```python
from build123d import *

# Parameters (mm, degrees)
S_BOX1_W       = 20
S_BOX1_H       = 2.5
BOSS_1_DEPTH   = 42
S_BOX2_W       = 30.4
S_BOX2_H       = 17
BOSS_2_DEPTH   = 27.6
S_CUT3_W       = 30.6
S_CUT3_H       = 13
POCKET_3_DEPTH = 23.6
S_HOLE4_R      = 1.5
HOLE_4_DEPTH   = 2.7


with BuildPart() as part:
    # S_box1 → Boss_1 (new body)
    with BuildSketch(Plane.XY.offset(-34)):
        with Locations((0, -2.75)):
            Rectangle(S_BOX1_W, S_BOX1_H)
    extrude(amount=BOSS_1_DEPTH)

    # S_box2 → Boss_2 (add)
    with BuildSketch(Plane.XY.offset(-35.4)):
        with Locations((-3.8, -10)):
            Rectangle(S_BOX2_W, S_BOX2_H)
    extrude(amount=BOSS_2_DEPTH)

    # S_cut3 → Pocket_3 (cut)
    with BuildSketch(Plane.XY.offset(-33.4)):
        with Locations((-3.8, -10)):
            Rectangle(S_CUT3_W, S_CUT3_H)
    extrude(amount=POCKET_3_DEPTH, mode=Mode.SUBTRACT)

    # S_hole4 → Hole_4 (cut)
    with BuildSketch(Plane(origin=(0, -4.1, 0), x_dir=(1, 0, 0), z_dir=(0, 1, 0))):
        with Locations(Location((0, 0, 0), (0, 0, 90))):
            Circle(S_HOLE4_R)
    extrude(amount=HOLE_4_DEPTH, mode=Mode.SUBTRACT)


solid = part.part
```
Geometry check sheet. Reference: the model listing, model coordinates, mm. A direction names the side the tool comes from. Round coordinates to 2 decimals unless told otherwise and drop trailing zeros. Loops run counter-clockwise (first coordinate to the right, second up) from the corner with the lowest first, then second, coordinate; pieces in that order, holes last. Notation, with made-up numbers: M 78,-40 L 136,-40 A17 ccw 136,-8 Z; hole C 25,27 d4. An arc over 180 degrees is marked long. Return JSON: item names as keys, results as strings. Group by question number.
(1) Scan lines: line 1 along X through (y, z) = (-2, 0); line 2 along Z through (x, y) = (6, -7); line 3 along Y through (x, z) = (1, -18). Record each from-to range of solid material in increasing order. Write a range as [from, to].
(2) Section check A-A, the plane x = 0. Enter the section's corners in (y, z).
(3) Go/stop test with flat-tipped pins: pin 1 (17.5 mm diameter, centred on x = -4, z = 3.5, fed in from -Y); pin 2 (5 mm diameter, centred on x = -8, y = -10, fed in from +Z); pin 3 (0.8 mm diameter, centred on y = -3, z = -1.5, fed in from -X). Record where each tip stops, or that it passes through.
(4) Set-up check for faces 5 (the face through (10, -3, 0)), 6 (the face through (0, -4, 2)), 7 (the face through (-4, -10, -33.4)): record each of +Z, -Z, +X, -X, +Y, -Y from which the full face is reachable in a straight line by a thin tool's end or side.
(5) Section check B-B, the plane z = -14. Enter the section's corners in (x, y).
(6) Section check C-C, the plane y = -12.75. Enter the section's corners in (x, z).
(7) Section check D-D, the plane x = 3.5. Enter the section's corners in (y, z).
(8) Mould release check, pull along Z, two halves, no side actions. Record for faces 1 (the face through (-4, -10, -35.4)), 2 (the face through (-10, -3, 0)), 3 (the face through (0, -3, 8)), 4 (the face through (-0.45, -2.77, -1.43)): pulls with the +Z half, pulls with the -Z half, needs draft (parallel to the pull), parting line crosses it, or undercut.
Data:
{
 "1": {"line 1": "[-10, -1.5], [1.5, 10]", "line 2": "[-35.4, -33.4], [-9.8, -7.8]", "line 3": "[-18.5, -16.5], [-3.5, -1.5]"},
 "2": {"outline": "M -18.5,-35.4 L -1.5,-35.4 L -1.5,-1.5 L -4,-1.5 L -4,-7.8 L -18.5,-7.8 Z; M -4,1.5 L -1.5,1.5 L -1.5,8 L -4,8 Z; hole M -16.5,-33.4 L -3.5,-33.4 L -3.5,-9.8 L -16.5,-9.8 Z"},
 "3": {"pin 1": "y = -4", "pin 2": "z = -7.8", "pin 3": "x = -10"},
 "4": {"face 5": "+Z, +X, +Y, -Y", "face 6": "+Z, +X, -X, -Y", "face 7": "+X, -X"},
 "5": {"outline": "M -19,-18.5 L 11.4,-18.5 L 11.4,-16.5 L -19,-16.5 Z; M -19,-3.5 L 11.4,-3.5 L 11.4,-1.5 L -19,-1.5 Z"},
 "6": {"outline": "M -19,-35.4 L 11.4,-35.4 L 11.4,-33.4 L -19,-33.4 Z; M -19,-9.8 L 11.4,-9.8 L 11.4,-7.8 L -19,-7.8 Z"},
 "7": {"outline": "M -18.5,-35.4 L -1.5,-35.4 L -1.5,8 L -4,8 L -4,-7.8 L -18.5,-7.8 Z; hole M -16.5,-33.4 L -3.5,-33.4 L -3.5,-9.8 L -16.5,-9.8 Z"},
 "8": {"face 1": "pulls with the -Z half", "face 2": "needs draft", "face 3": "pulls with the +Z half", "face 4": "undercut"}
}
